```python
from build123d import *

# Parameters (mm, degrees)
PAD005_DEPTH = 12.5
PAD006_DEPTH = 10
PAD007_DEPTH = 10
SKETCH012_W  = 415
SKETCH012_H  = 16
PAD008_DEPTH = 8


with BuildPart() as part:
    # Sketch008 → Pad005 (new body, symmetric)
    with BuildSketch(Plane.YZ):
        Polygon((-235, 194), (235, 194), (235, 185), (207.5, 185), (207.5, 176), (-207.5, 176), (-207.5, 185), (-235, 185), align=None)
    extrude(amount=PAD005_DEPTH, both=True)

    # Sketch010 (on Face6 of Pad005) → Pad006 (join)
    with BuildSketch(Plane(origin=(0, -207.5, 0), x_dir=(0, 0, -1), z_dir=(0, -1, 0))):
        Polygon((-185, 18), (-185, -18), (-115, -18), (-109.5, -12.5), (-4, -12.5), (-4, 12.5), (-109.5, 12.5), (-115, 18), align=None)
    extrude(amount=PAD006_DEPTH)

    # Sketch011 (on Face8 of Pad006) → Pad007 (join)
    with BuildSketch(Plane.ZX.offset(207.5)):
        Polygon((4, 12.5), (109.5, 12.5), (115, 18), (185, 18), (185, -18), (115, -18), (109.5, -12.5), (4, -12.5), align=None)
    extrude(amount=PAD007_DEPTH)

    # Sketch012 → Pad008 (join, symmetric)
    with BuildSketch(Plane.YZ):
        with Locations((0, 12)):
            Rectangle(SKETCH012_W, SKETCH012_H)
    extrude(amount=PAD008_DEPTH, both=True)


solid = part.part
```
Source: CAD feature listing. Evaluate the final solid. Frame: model axes, mm. A direction names the side the tool comes from. Round coordinates to 2 decimals unless told otherwise and drop trailing zeros. Write each loop counter-clockwise with the first axis right and the second up, starting at its lowest first coordinate (ties: lowest second). Pieces come first, ordered by that corner, then holes. Notation, with made-up numbers: M 7.5,42 L 39.5,42 A19 cw 39.5,60 Z; hole C -33.75,-17 d3. An arc over 180 degrees is marked long. Answer as a JSON object with one key per item and string values. Group by question number.
(1) Section query A-A on x = 3. Output: boundary loops of the cut face in (y, z), then the cut area to 3 significant figures.
(2) Section query B-B on z = 125. Output: boundary loops of the cut face in (x, y).
(3) Reachability of faces 1 (the flat face through (-12.5, -212, 57)), 2 (the flat face through (0, 226, 185)), 3 (the flat face through (-8, -3, 12)) from +Z, -Z, +X, -X, +Y, -Y: full face, straight path, thin tool, end or side. Return the list, or none.
(4) First-contact query: pin 1 (18 mm diameter, centred on x = 0.5, z = 129, fed in from +Y); pin 2 (3 mm diameter, centred on x = 14.5, y = -212, fed in from +Z); pin 3 (8 mm diameter, centred on y = -42, z = 11, fed in from -X). Flat tips, straight axial feed; report the tip coordinate or a pass-through.
(5) Section query C-C on y = -74.5. Output: boundary loops of the cut face in (x, z), then the cut area to 3 significant figures.
(6) Ray query, line 1 (Y direction, x = -5.5, z = 138.5); line 2 (Z direction, x = 1, y = 203); line 3 (X direction, y = 109, z = 179). Return the intervals inside material, ascending. Write a range as [from, to].
(7) Mould query, pull axis Y, two halves, no side actions, for faces 4 (the flat face through (18, 212, 150)), 5 (the flat face through (8, -3, 12)), 6 (the flat face through (0, 235, 190)), 7 (the flat face through (0, -217.5, 96)). Classes: +Y half, -Y half, draft (parallel to the pull), parting line (faces both ways), or undercut.
Computed values:
{
 "1": {"outline": "M -235,185 L -217.5,185 L -217.5,4 L 217.5,4 L 217.5,185 L 235,185 L 235,194 L -235,194 Z; hole M -207.5,20 L 207.5,20 L 207.5,176 L -207.5,176 Z", "area": "18,200 mm^2"},
 "2": {"outline": "M -18,-217.5 L 18,-217.5 L 18,-207.5 L -18,-207.5 Z; M -18,207.5 L 18,207.5 L 18,217.5 L -18,217.5 Z"},
 "3": {"face 1": "-Z, -X, +Y, -Y", "face 2": "-Z, +X, -X, +Y", "face 3": "-Z, -X"},
 "4": {"pin 1": "y = 217.5", "pin 2": "z = 185", "pin 3": "x = -8"},
 "5": {"outline": "M -12.5,176 L 12.5,176 L 12.5,194 L -12.5,194 Z; M -8,4 L 8,4 L 8,20 L -8,20 Z", "area": "706 mm^2"},
 "6": {"line 1": "[-217.5, -207.5], [207.5, 217.5]", "line 2": "[4, 20], [176, 194]", "line 3": "[-12.5, 12.5]"},
 "7": {"face 4": "draft", "face 5": "undercut", "face 6": "+Y half", "face 7": "-Y half"}
}
